```python
from build123d import *

# Parameters (mm, degrees)
F0_W      = 73
F0_H      = 73
F1_DEPTH  = 25
F2_R      = 5
F3_R      = 27.5
F4_DEPTH  = 3
F5_R      = 2.4
F6_DEPTH  = 4
F7_SIZE   = 1
F9_W      = 110.5126142502
F9_H      = 98.0203673244
F10_DEPTH = 40.1
F14_D     = 5


# Not quite as in the source:
# - a feature of the source that left no trace in its solid (it failed there, or was rolled back) is left out


with BuildPart() as f1:
    # F0 (on Top) → F1 (new body)
    with BuildSketch(Plane.XY):
        Rectangle(F0_W, F0_H)
    extrude(amount=F1_DEPTH)

    # F2
    f2_edges = [f1.edges().sort_by_distance(p)[0] for p in [
        (0, 36.5, 25),
        (0, -36.5, 25),
        (36.5, 0, 25),
        (-36.5, 0, 25),
    ]]
    fillet(f2_edges, radius=F2_R)

    # F3 (on face) → F4 (cut)
    with BuildSketch(Plane.XY.offset(25)):
        Circle(F3_R)
    extrude(amount=-F4_DEPTH, mode=Mode.SUBTRACT)

    # F5 (on face) → F6 (join)
    with BuildSketch(Plane.XY):
        with Locations((-23.6, -32.1)):
            Circle(F5_R)
        with Locations((23.6, -32.1)):
            Circle(F5_R)
        with Locations((-23.6, 32.1)):
            Circle(F5_R)
        with Locations((23.6, 32.1)):
            Circle(F5_R)
    extrude(amount=-F6_DEPTH)

    # F7
    f7_edges = [f1.edges().sort_by_distance(p)[0] for p in [
        (-26, -32.1, -4),
        (-26, 32.1, -4),
        (21.2, 32.1, -4),
        (21.2, -32.1, -4),
    ]]
    chamfer(f7_edges, length=F7_SIZE)

    # F14 (through all)
    with Locations(Plane.XY.offset(22)):
        with Locations((0, 0)):
            Hole(F14_D / 2)


with BuildPart() as f10:
    # F9 (on offset) → F10 (new body, through all)
    with BuildSketch(Plane.XY.offset(40.1)):
        Rectangle(F9_W, F9_H)
    extrude(amount=-F10_DEPTH)


solid = f1.part
```
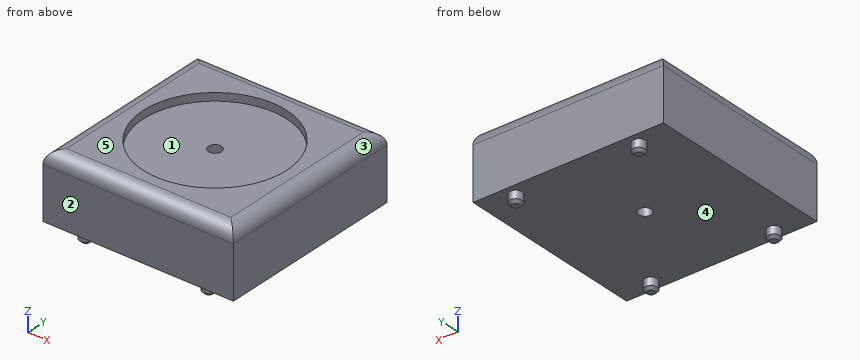
The listing builds one solid part. Answer for the finished solid, in the listing's coordinates (mm). Face numbers are marked on the shaded views. A direction names the side the tool comes from. Round coordinates to 2 decimals unless told otherwise and drop trailing zeros. Write each loop counter-clockwise with the first axis right and the second up, starting at its lowest first coordinate (ties: lowest second). Pieces come first, ordered by that corner, then holes. Notation, with made-up numbers: (67.25, 47.5) -> (75.25, 47.5) arc R20 ccw to (75.25, 58.5) -> close; hole circle Ø2 at (-26, 49). An arc over 180 degrees is marked (long way). Write item = value, one per line.
1) Section A-A on x = 0 is taken. Write down the section's boundary in (y, z).
Check values:
outline = (-36.5, 0) -> (-2.5, 0) -> (-2.5, 22) -> (-27.5, 22) -> (-27.5, 25) -> (-31.5, 25) arc R5 ccw to (-36.5, 20) -> close; (2.5, 0) -> (36.5, 0) -> (36.5, 20) arc R5 ccw to (31.5, 25) -> (27.5, 25) -> (27.5, 22) -> (2.5, 22) -> close
2) For a pull along Y with two mould halves and no side action, classify the marked faces 1, 2 and 3 as released by +Y, released by -Y, zero draft, split by the parting line, or undercut.
Check values:
face_1 = undercut
face_2 = released by -Y
face_3 = zero draft
3) Given pin 1 (16.5 mm diameter, centred on x = 8.5, y = -10, fed in from +Z); pin 2 (6 mm diameter, centred on x = 0, y = 0, fed in from -Z), each flat-ended and moving along its own axis, determine where each tip first touches the part or whether it passes through.
Check values:
pin_1 = 22
pin_2 = 0
4) Which of the six approach directions +Z, -Z, +X, -X, +Y, -Y give full straight-line access (tool end or side, diameter ignored) to the marked faces 4 and 5?
Check values:
face_4 = -Z
face_5 = +Z, +X, -X, +Y, -Y
5) Section C-C on x = 23.6 is taken. Write down the section's boundary in (y, z).
Check values:
outline = (-36.5, 0) -> (-34.5, 0) -> (-34.5, -3) -> (-33.5, -4) -> (-30.7, -4) -> (-29.7, -3) -> (-29.7, 0) -> (29.7, 0) -> (29.7, -3) -> (30.7, -4) -> (33.5, -4) -> (34.5, -3) -> (34.5, 0) -> (36.5, 0) -> (36.5, 20) arc R5 ccw to (31.5, 25) -> (14.12, 25) -> (14.12, 22) -> (-14.12, 22) -> (-14.12, 25) -> (-31.5, 25) arc R5 ccw to (-36.5, 20) -> close
6) Straight lines are drawn through the part: line 1 along Y through (x, z) = (0, 5); line 2 along Z through (x, y) = (-23.5, 2); line 3 along Y through (x, z) = (0, 24.1). For each, find the intervals that lie inside material, in ascending order. Write a range as [from, to].
Check values:
line_1 = [-36.5, -2.5], [2.5, 36.5]
line_2 = [0, 22]
line_3 = [-34.36, -27.5], [27.5, 34.36]
7) Section D-D on y = 18 is taken. Write down the section's boundary in (x, z), plus the area to 3 significant figures.
Check values:
outline = (-36.5, 0) -> (36.5, 0) -> (36.5, 20) arc R5 ccw to (31.5, 25) -> (20.79, 25) -> (20.79, 22) -> (-20.79, 22) -> (-20.79, 25) -> (-31.5, 25) arc R5 ccw to (-36.5, 20) -> close
area = 1,690 mm²
